Input: part model. Units: mm. Frame: model coordinates. A direction names the side the tool comes from. Coordinates: 2 decimals unless noted, no trailing zeros. Write each loop counter-clockwise with the first axis right and the second up, starting at its lowest first coordinate (ties: lowest second). Pieces come first, ordered by that corner, then holes.
1) Line query: L1, parallel to X at y = 4, z = -29; L2, parallel to Z at x = -119.5, y = 0.5; L3, parallel to X at y = 1.25, z = -19.5. Output: solid intervals per line, ascending.
2) Section query A-A (y = 1). Output: boundary loops of the cut face in (x, z) (3 decimals), then the cut area to 3 significant figures.
3) Set-up query: faces 1 (the flat face through (-143, 1, -22.356)), 2 (the flat face through (-34, 5, -24.781)), 3 (the cylindrical face through (-133.047, 4.958, -19.402)), 4 (the flat face through (-34, 1, -16.206)). Return all of +Z, -Z, +X, -X, +Y, -Y with unobstructed straight access to the full face (end or side cutting, diameter ignored); none if empty.
4) Draft query along Z for faces 5 (the flat face through (-89, 4, -32.781)), 6 (the flat face through (-37, 2, -23)), 7 (the flat face through (-88, 8, -19)). Return one class per face: pulls with the +Z half, pulls with the -Z half, needs draft (parallel to the pull), parting line crosses it, or undercut.
5) Pin query (flat end, axial travel): pin 1 Ø3.5 at (x, z) = (-141, -21) entering from +Y. Return the tip coordinate at first contact, or that it passes through.
Autodesk Inventor part; units mm, degrees
ref_plane "YZ Plane" through (0, 0, 0) normal (1, 0, 0) x (0, 1, 0)
ref_plane "XZ Plane" through (0, 0, 0) normal (0, 1, 0) x (-1, 0, 0)
ref_plane "XY Plane" through (0, 0, 0) normal (0, 0, 1) x (1, 0, 0)
sketch "Sketch1" plane through (0, 0, 0) normal (0, 1, 0) x (-1, 0, 0)
  circle A0 centre (118.5461, -28.7809) radius 1.975
  circle A1 centre (118.5461, -9.7809) radius 1.975
  arc A2 (138.5461, -13.7809) -> (138.5461, -24.7809) centre (138.5461, -19.2809) ccw
  circle A3 centre (58.5461, -28.8073) radius 1.975
  line L0 (147.5461, -32.7809) -> (29.5461, -32.7809)
  line L1 (29.5461, -5.7809) -> (147.5461, -5.7809)
  arc A4 (38.5461, -24.7809) -> (38.5461, -13.7809) centre (38.5461, -19.2809) ccw
  line L2 (29.5461, -32.7809) -> (29.5461, -5.7809)
  circle A5 centre (58.5461, -9.8073) radius 1.975
  arc A6 (138.5461, -16.2059) -> (138.5461, -22.3559) centre (138.5461, -19.2809) ccw
  arc A7 (38.5461, -22.3559) -> (38.5461, -16.2059) centre (38.5461, -19.2809) ccw
  line L3 (143.1062, -22.3559) -> (147.5461, -22.3559)
  line L4 (143.1062, -16.2059) -> (147.5461, -16.2059)
  line L5 (147.5461, -32.7809) -> (147.5461, -22.3559)
  line L6 (147.5461, -16.2059) -> (147.5461, -5.7809)
  line L7 (143.1062, -22.3559) -> (138.5461, -22.3559)
  line L8 (143.1062, -16.2059) -> (138.5461, -16.2059)
  line L9 (138.5461, -24.7809) -> (147.5461, -24.7809)
  line L10 (138.5461, -13.7809) -> (147.5461, -13.7809)
  line L11 (38.5461, -22.3559) -> (29.5461, -22.3559)
  line L12 (38.5461, -24.7809) -> (29.5461, -24.7809)
  line L13 (38.5461, -16.2059) -> (29.5461, -16.2059)
  line L14 (38.5461, -13.7809) -> (29.5461, -13.7809)
  point P0 (88.5461, -32.7809)
  point P1 (88.5461, -5.7809)
  dimension "d162" = 60
  dimension "d163" = 60
  dimension "d165" = 100
  dimension "d183" = 11
  dimension "d184" = 11
  dimension "d185" = 6.15
  dimension "d186" = 6.15
  dimension "d187" = 3.95
  dimension "d188" = 3.95
  dimension "d189" = 3.95
  dimension "d190" = 3.95
  dimension "d202" = 9
  dimension "d203" = 9
  dimension "d204" = 9
  dimension "d212" = 19
  dimension "d213" = 19
  dimension "d214" = 27
  dimension "d215" = 4
  dimension "d216" = 4
  dimension "d217" = 13.5
  dimension "d218" = 30
  dimension "d219" = 30
extrude "Extrusion13" add sketch "Sketch1" along normal blind 8 contours A2 L9 L5 L0 L2 L12 A4 L14 L1 L6 L10
extrude "Extrusion14" add sketch "Sketch1" along normal blind 2 contours L14 A4 L12 L2 L11 A7 L13
extrude "Extrusion15" add sketch "Sketch1" along normal blind 2 contours L10 L6 L4 L8 A6 L7 L3 L5 L9 A2
properties part number "Base Laser_3DPrint"
Answer:
1. L1: x = -147.55 to -120.51, -116.58 to -60.51, -56.58 to -29.55
1. L2: z = -32.78 to -30.51, -27.05 to -11.51, -8.05 to -5.78
1. L3: x = -135.48 to -41.61
2. outline: (-147.546, -32.781) - (-29.546, -32.781) - (-29.546, -22.356) - (-38.546, -22.356) arc R3.075 cw to (-38.546, -16.206) - (-29.546, -16.206) - (-29.546, -5.781) - (-147.546, -5.781) - (-147.546, -16.206) - (-138.546, -16.206) arc R3.075 cw to (-138.546, -22.356) - (-147.546, -22.356) - close; hole circle Ø3.95 at (-118.546, -28.781); hole circle Ø3.95 at (-118.546, -9.781); hole circle Ø3.95 at (-58.546, -28.807); hole circle Ø3.95 at (-58.546, -9.807)
2. area: 3,000 mm2
3. face 1: -X, +Y, -Y
3. face 2: +X, +Y
3. face 3: -X, +Y
3. face 4: +X, +Y, -Y
4. face 5: pulls with the -Z half
4. face 6: undercut
4. face 7: needs draft
5. pin 1: stops at y = 2
